Here's how the part is built. I have some questions about the finished solid (model axes, mm). A direction names the side the tool comes from. Round coordinates to 2 decimals unless told otherwise and drop trailing zeros. Loops run counter-clockwise (first coordinate to the right, second up) from the corner with the lowest first, then second, coordinate; pieces in that order, holes last. Notation, with made-up numbers: M -36,77 L -10,77 A26 ccw -10,95 Z; hole C 47.5,-20.5 d7. An arc over 180 degrees is marked long. Use a Markdown table: item, result.
```python
from build123d import *

# Parameters (mm, degrees)
F1_DEPTH = 88.9
F2_R     = 21.59
F3_DEPTH = 76.2
F4_W     = 38.340382
F4_H     = 35.473824
F4_W_2   = 37.265419
F4_H_2   = 36.548784
F5_DEPTH = 12.7
F6_R     = 5.08


with BuildPart() as f1:
    # F0 (on Top) → F1 (new body)
    with BuildSketch(Plane.XY):
        with BuildLine():
            ThreePointArc((-75.779863, 38.1), (-64.620631, 11.159232), (-37.679863, 0))
            Line((-37.679863, 0), (124.880137, 0))
            ThreePointArc((124.880137, 0), (151.820906, 11.159232), (162.980137, 38.1))
            Line((162.980137, 38.1), (162.980137, 86.36))
            ThreePointArc((162.980137, 86.36), (151.820906, 113.300768), (124.880137, 124.46))
            Line((124.880137, 124.46), (-37.679863, 124.46))
            ThreePointArc((-37.679863, 124.46), (-64.620631, 113.300768), (-75.779863, 86.36))
            Line((-75.779863, 86.36), (-75.779863, 38.1))
        make_face()
    extrude(amount=F1_DEPTH)

    # F2 (on face) → F3 (cut)
    with BuildSketch(Plane.YZ.offset(162.980137)):
        with Locations((38.1, 47.477592)):
            Circle(F2_R)
        with Locations((86.36, 47.182769)):
            Circle(F2_R)
    extrude(amount=-F3_DEPTH, mode=Mode.SUBTRACT)

    # F4 (on face) → F5 (join)
    with BuildSketch(Plane.XY.offset(88.9)):
        with Locations((115.770999, 93.28603)):
            Rectangle(F4_W, F4_H)
        with Locations((116.308481, 35.058801)):
            Rectangle(F4_W_2, F4_H_2)
    extrude(amount=F5_DEPTH)

    # F6
    f6_edges = [f1.edges().sort_by_distance(p)[0] for p in [
        (115.770999, 111.022942, 101.6),
        (96.600808, 93.28603, 101.6),
        (115.770999, 75.549118, 101.6),
        (134.94119, 93.28603, 101.6),
        (116.308481, 53.333193, 101.6),
        (97.675771, 35.058801, 101.6),
        (116.308481, 16.784409, 101.6),
        (134.94119, 35.058801, 101.6),
    ]]
    fillet(f6_edges, radius=F6_R)


solid = f1.part
```
Q1. I need wall thicknesses on line 1 (Z direction, x = 109.5, y = 38.1); line 2 (Z direction, x = -35.5, y = 30.5); line 3 (X direction, y = 30, z = 96.5). Which ranges of each line are inside material? Lowest first, please. Write a range as from..to.
Return value:
| item | result |
|---|---|
| line 1 | z = 0..25.89, 69.07..101.6 |
| line 2 | z = 0..88.9 |
| line 3 | x = 97.68..134.94 |
Q2. We'd pull the mould along Y, two halves only. Please class faces 6 (the flat face through (42, 0, 44)), 7 (the cylindrical face through (116.569, 51.885, 100.072)), 8 (the cylindrical face through (133.493, 93.534, 100.072)): pulls with the +Y half, pulls with the -Y half, needs draft (parallel to the pull), parting line crosses it, or undercut.
Return value:
| item | result |
|---|---|
| face 6 | pulls with the -Y half |
| face 7 | undercut |
| face 8 | needs draft |
Q3. Imagine slicing it at A-A, the plane z = 9.5. Please give me the cut outline in (x, y), then the cut area to 3 significant figures.
Return value:
| item | result |
|---|---|
| outline | M -75.78,38.1 A38.1 ccw -37.68,0 L 124.88,0 A38.1 ccw 162.98,38.1 L 162.98,86.36 A38.1 ccw 124.88,124.46 L -37.68,124.46 A38.1 ccw -75.78,86.36 Z |
| area | 28,500 mm^2 |
Q4. Imagine slicing it at B-B, the plane y = 27. Please give me the cut outline in (x, z), then the cut area to 3 significant figures.
Return value:
| item | result |
|---|---|
| outline | M -74.13,0 L 161.33,0 L 161.33,28.96 L 86.78,28.96 L 86.78,66 L 161.33,66 L 161.33,88.9 L 134.94,88.9 L 134.94,96.52 A5.08 ccw 129.86,101.6 L 102.76,101.6 A5.08 ccw 97.68,96.52 L 97.68,88.9 L -74.13,88.9 Z |
| area | 18,600 mm^2 |
Q5. Will these pins go through, and if not, where does the flat tip stop? P1, Ø6, axis at y = 36.5, z = 92.5, coming from the +X side; P2, Ø4, axis at y = 92.5, z = 93, coming from the -X side; P3, Ø4, axis at x = 122, z = 93.5, coming from the +Y side.
Return value:
| item | result |
|---|---|
| P1 | stops at x = 134.94 |
| P2 | stops at x = 96.6 |
| P3 | stops at y = 111.02 |
Q6. For faces 1 (the cylindrical face through (116.039, 76.998, 100.072)), 2 (the flat face through (97.676, 35, 93)), 3 (the flat face through (134.941, 93, 93)), 4 (the flat face through (96.601, 93, 93)), 5 (the flat face through (116, 16.784, 93)), which set-ups out of +Z, -Z, +X, -X, +Y, -Y let a thin tool reach every point of the face, with its end or its side?
Return value:
| item | result |
|---|---|
| face 1 | +Z, +X, -X |
| face 2 | +Z, -X, -Y |
| face 3 | +Z, +X, +Y, -Y |
| face 4 | +Z, -X, +Y, -Y |
| face 5 | +Z, +X, -X, -Y |
Q7. Imagine slicing it at D-D, the plane z = 43.5. Please give me the cut outline in (x, y).
Return value:
| item | result |
|---|---|
| outline | M -75.78,38.1 A38.1 ccw -37.68,0 L 124.88,0 A38.1 ccw 156.52,16.88 L 86.78,16.88 L 86.78,59.32 L 162.98,59.32 L 162.98,65.09 L 86.78,65.09 L 86.78,107.63 L 156.49,107.63 A38.1 ccw 124.88,124.46 L -37.68,124.46 A38.1 ccw -75.78,86.36 Z |
Q8. Imagine slicing it at C-C, the plane x = -8. Please give me the cut outline in (y, z), then the cut area to 3 significant figures.
Return value:
| item | result |
|---|---|
| outline | M 0,0 L 124.46,0 L 124.46,88.9 L 0,88.9 Z |
| area | 11,100 mm^2 |
